```python
from build123d import *

# Parameters (mm, degrees)
SKETCH_1_R          = 1.5
EXTRUDE_1_DEPTH     = 2
SKETCH_2_W          = 2
SKETCH_2_H          = 4
EXTRUDE_5_DEPTH     = 18
SKETCH_5_W          = 3
SKETCH_5_H          = 2
EXTRUDE_6_DEPTH     = 35
SKETCH_7_W          = 2
SKETCH_7_H          = 4
EXTRUDE_9_DEPTH     = 8
SKETCH_9_W          = 10
SKETCH_9_H          = 31
CUT_EXTRUDE_2_DEPTH = 15
SKETCH_10_W         = 3
SKETCH_10_H         = 31
EXTRUDE_10_DEPTH    = 2
FILLET_1_R          = 8


with BuildPart() as part:
    # 草图1 → 凸台-拉伸1 (new body)
    with BuildSketch(Plane.XY):
        with BuildLine():
            Line((5, 60), (5, -60))
            ThreePointArc((5, -60), (0, -65), (-5, -60))
            Line((-5, -60), (-5, 60))
            ThreePointArc((-5, 60), (0, 65), (5, 60))
        make_face()
        with Locations((0, 60)):
            Circle(SKETCH_1_R, mode=Mode.SUBTRACT)
        with Locations(Location((0, -60, 0), (0, 0, 180))):
            Circle(SKETCH_1_R, mode=Mode.SUBTRACT)
        Circle(SKETCH_1_R, mode=Mode.SUBTRACT)
    extrude(amount=EXTRUDE_1_DEPTH)

    # 草图2 → 凸台-拉伸5 (add)
    with BuildSketch(Plane.ZY.offset(5)):
        with Locations((1, 55)):
            Rectangle(SKETCH_2_W, SKETCH_2_H)
    extrude(amount=-EXTRUDE_5_DEPTH)

    # 草图5 → 凸台-拉伸6 (add)
    with BuildSketch(Plane.XZ.offset(-53)):
        with Locations((11.5, 1)):
            Rectangle(SKETCH_5_W, SKETCH_5_H)
    extrude(amount=EXTRUDE_6_DEPTH)

    # 草图7 → 凸台-拉伸9 (add)
    with BuildSketch(Plane(origin=(13, 0, 0), x_dir=(0, 0, -1), z_dir=(1, 0, 0))):
        with Locations((-1, 20)):
            Rectangle(SKETCH_7_W, SKETCH_7_H)
    extrude(amount=-EXTRUDE_9_DEPTH)

    # 草图9 → 切除-拉伸2 (cut)
    with BuildSketch(Plane(origin=(0, 0, 0), x_dir=(-1, 0, 0), z_dir=(0, 0, -1))):
        with Locations((0, 37.5)):
            Rectangle(SKETCH_9_W, SKETCH_9_H)
    extrude(amount=-CUT_EXTRUDE_2_DEPTH, mode=Mode.SUBTRACT)

    # 草图10 → 凸台-拉伸10 (add)
    with BuildSketch(Plane(origin=(0, 0, 0), x_dir=(-1, 0, 0), z_dir=(0, 0, -1))):
        with Locations((-8.5, 37.5)):
            Rectangle(SKETCH_10_W, SKETCH_10_H)
    extrude(amount=-EXTRUDE_10_DEPTH)

    # 圆角1
    # the kernel refuses this fillet: 8 mm, written as the material it takes off along each edge
    with BuildSketch(Plane(origin=(-5, 53, -19.843134833), x_dir=(1, 0, 0), z_dir=(0, 0, 1))) as fillet_1_piece_1:
        with BuildLine():
            CenterArc((7.937253933, 8), FILLET_1_R, 187.180755781, 82.819244219)
            Line((0, 7), (0, 0))
            Line((0, 0), (7.937253933, 0))
        make_face()
    extrude(amount=41.686269666, mode=Mode.SUBTRACT)


solid = part.part
```
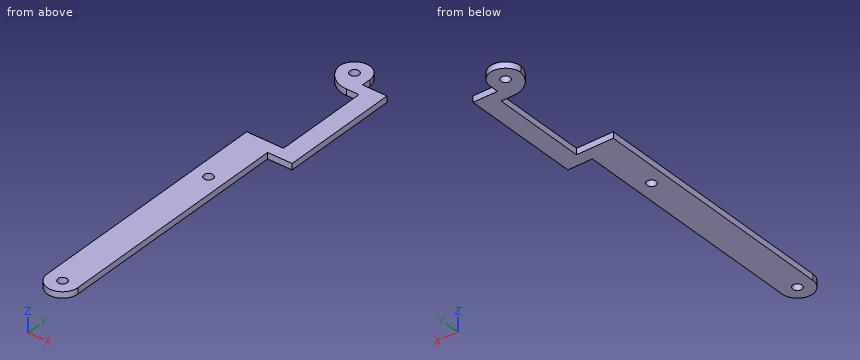
Verification items for the finished model (mm, model axes). Coordinates: 2 decimals unless noted, no trailing zeros. Write each loop counter-clockwise with the first axis right and the second up, starting at its lowest first coordinate (ties: lowest second). Pieces come first, ordered by that corner, then holes. Notation, with made-up numbers: (-2, -2.5) - (31, -2.5) arc R29 ccw to (31, 26.5) - close; hole circle Ø8 at (58, 32). An arc over 180 degrees is marked (long way). One line per question, with ' | ' between items. Start each with the question number.
1. Gauge pin test, flat ends, axial feed: P1, Ø0.6, axis at x = 7, z = 1, coming from the +Y side; P2, Ø0.6, axis at x = 7, z = 1, coming from the -Y side; P3, Ø1, axis at x = 1, z = 2, coming from the +Y side. Record the tip position at first contact, or that the pin passes through.
2. Section check D-D (x = 11). Enter the section's corners in (y, z), plus the area to 3 significant figures.
3. Material ranges on line 1 along X through (y, z) = (-60, 0.5); line 2 along Y through (x, z) = (5.5, 1); line 3 along Y through (x, z) = (0, 0.8), recorded low to high.
4. Section check B-B (z = 0.3). Enter the section's corners in (x, y).
5. Section check A-A (y = 0). Enter the section's corners in (x, z), plus the area to 3 significant figures.
6. Section check C-C (x = 0). Enter the section's corners in (y, z), plus the area to 3 significant figures.
Computed values:
1) P1: y = 57 | P2: y = 18 | P3: y = 64.97
2) outline: (18, 0) - (57, 0) - (57, 2) - (18, 2) - close | area: 78.0 mm²
3) line 1: -5 to -1.5, 1.5 to 5 | line 2: 18 to 22, 53 to 57 | line 3: -65 to -61.5, -58.5 to -1.5, 1.5 to 22, 53.56 to 58.5, 61.5 to 65
4) outline: (-5, -60) arc R5 ccw to (5, -60) - (5, 18) - (13, 18) - (13, 57) - (5, 57) - (5, 60) arc R5 ccw to (-5, 60) arc R8 ccw to (2.94, 53) - (7, 53) - (7, 22) - (-5, 22) - close; hole circle Ø3 at (0, -60); hole circle Ø3 at (0, 0); hole circle Ø3 at (0, 60)
5) outline: (-5, 0) - (-1.5, 0) - (-1.5, 2) - (-5, 2) - close; (1.5, 0) - (5, 0) - (5, 2) - (1.5, 2) - close | area: 14.0 mm²
6) outline: (-65, 0) - (-61.5, 0) - (-61.5, 2) - (-65, 2) - close; (-58.5, 0) - (-1.5, 0) - (-1.5, 2) - (-58.5, 2) - close; (1.5, 0) - (22, 0) - (22, 2) - (1.5, 2) - close; (53.56, 0) - (58.5, 0) - (58.5, 2) - (53.56, 2) - close; (61.5, 0) - (65, 0) - (65, 2) - (61.5, 2) - close | area: 179 mm²
